For this review, take the finished solid that the model builds, in its own axes (mm). Face numbers are marked on the shaded views. A direction names the side the tool comes from. Coordinates: 2 decimals unless noted, no trailing zeros. Write each loop counter-clockwise with the first axis right and the second up, starting at its lowest first coordinate (ties: lowest second). Pieces come first, ordered by that corner, then holes. Notation, with made-up numbers: (63, 0.5) - (98, 0.5) arc R18 cw to (98, 17.5) - close; hole circle Ø7 at (5.25, 71.5). An arc over 180 degrees is marked (long way). Write each question's results on one line, items separated by ' | '.
from build123d import *

# Parameters (mm, degrees)
PAD_DEPTH = 27.5


with BuildPart() as part:
    # Sketch → Pad (new body)
    with BuildSketch(Plane.XY):
        with BuildLine():
            Line((0, 0), (0, 10.0498))
            Line((0, 10.0498), (3, 10.0498))
            Line((3, 10.0498), (3, -2.1002))
            ThreePointArc((2.019976, -3.1), (2.714134, -2.800208), (3, -2.1002))
            Line((2.019976, -3.1), (-18, -3.5))
            Line((-18, -3.5), (-18, 0))
            Line((-18, 0), (0, 0))
        make_face()
    extrude(amount=PAD_DEPTH)


solid = part.part
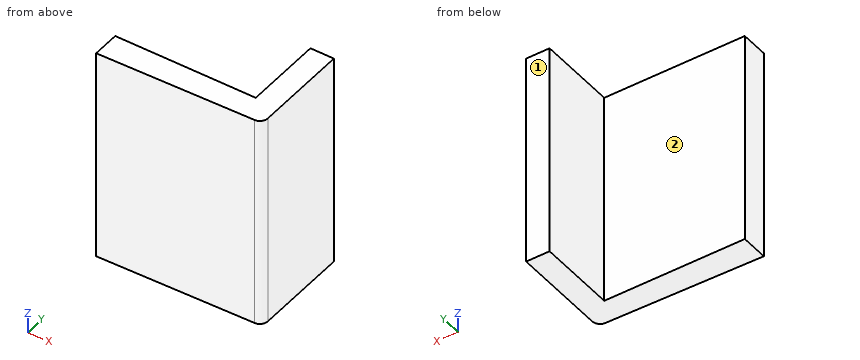
Q1. Take a section at A-A on z = 20.75. State the section outline as (x, y) points, plus the area to 3 significant figures.
Results found:
outline: (-18, -3.5) - (2.02, -3.1) arc R1 ccw to (3, -2.1) - (3, 10.05) - (0, 10.05) - (0, 0) - (-18, 0) - close | area: 99.0 mm2
Q2. Take a section at C-C on x = -9.25. State the section outline as (y, z) points.
Results found:
outline: (-3.33, 0) - (0, 0) - (0, 27.5) - (-3.33, 27.5) - close
Q3. Wall thickness on line 1 along Y through (x, z) = (2, 1); line 2 along X through (y, z) = (7.25, 20); line 3 along Y through (x, z) = (-17, 11): over which ranges is each line inside the solid? List them lowest first. Write a range as from..to.
Results found:
line 1: -3.1..10.05 | line 2: 0..3 | line 3: -3.48..0
Q4. Take a section at B-B on y = 3.5. State the section outline as (x, z) points.
Results found:
outline: (0, 0) - (3, 0) - (3, 27.5) - (0, 27.5) - close
Q5. For the marked faces 1 and 2, list the 3-axis set-ups (+Z, -Z, +X, -X, +Y, -Y) from which the entire face can be reached by the end or side of a thin tool; tool diameter is ignored.
Results found:
face 1: +Z, -Z, +X, -X, +Y | face 2: +Z, -Z, -X, +Y
Q6. For pin 1 (1 mm diameter, centred on x = -3.5, z = 7.5, fed in from +Y); pin 2 (5 mm diameter, centred on x = -5.5, y = -1.5, fed in from -Z); pin 3 (1 mm diameter, centred on y = 3, z = 13.5, fed in from -X); pin 4 (2 mm diameter, centred on x = -10, z = 5, fed in from -Y), all flat-tipped, find the tip position at first contact; note any pin that passes through.
Results found:
pin 1: y = 0 | pin 2: z = 0 | pin 3: x = 0 | pin 4: y = -3.36
